Model file for the job. Use its own axes, mm. A direction names the side the tool comes from. Coordinates: 2 decimals unless noted, no trailing zeros. Order: outer loops, then holes, each group sorted by start corner. A loop starts at its lowest first (then second) coordinate and runs counter-clockwise, first axis right, second up. Notation, with made-up numbers: (34.25, 31) -> (80.25, 31) arc R14 ccw to (80.25, 41) -> close; hole circle Ø6 at (58, -29.75). An arc over 180 degrees is marked (long way). Use CSV: the item, a comma, the result in double quotes. Start each with the question number.
(1) Pin check, flat tips, straight feed: pin 1 Ø1.6 at (y, z) = (0, 7.5) entering from -X; pin 2 Ø1 at (x, y) = (-5, -0.5) entering from -Z; pin 3 Ø1.5 at (x, y) = (-21, 0.5) entering from -Z. Stop position of each tip, or through.
(2) Cut at B-B on z = -8. Write the cut outline in (x, y), plus the area to 3 significant figures.
(3) Pull direction X, two halves, no side cores. Call faces 1 (the flat face through (-31, 0, 36.82)), 2 (the flat face through (-38, 0, -33.846)), 3 (the flat face through (-40, 0, 37)): pulls with the +X half, pulls with the -X half, needs draft (parallel to the pull), parting line crosses it, or undercut.
(4) Cut at A-A on x = 20. Write the cut outline in (y, z).
(5) Probe L1, parallel to Z at x = 16.5, y = 0.2. List the from-to ranges inside material, lowest first.
(6) Tool access for faces 4 (the flat face through (-36.82, 0, 6)), 5 (the flat face through (36.82, 0, 31)), 6 (the flat face through (-27.692, 0, 38)), 7 (the flat face through (-18, 0, -36.82)), 8 (the flat face through (0, 0, -40)): list every direction of +Z, -Z, +X, -X, +Y, -Y with a clear straight run to the whole face (end or side of a thin tool).
```python
from build123d import *

# Parameters (mm, degrees)
SKETCH1_W           = 80
SKETCH1_H           = 80
BOSS_EXTRUDE1_DEPTH = 1.5875
SKETCH2_OUTSIDE_W   = 104.636
SKETCH2_OUTSIDE_H   = 104.636
CUT_EXTRUDE1_DEPTH  = 57.657573413


with BuildPart() as part:
    # Sketch1 → Boss-Extrude1 (new, symmetric)
    with BuildSketch(Plane(origin=(0, 0, 0), x_dir=(1, 0, 0), z_dir=(0, 1, 0))):
        Rectangle(SKETCH1_W, SKETCH1_H)
    extrude(amount=BOSS_EXTRUDE1_DEPTH, both=True)

    # Sketch2 outside → Cut-Extrude1 (cut, through all)
    with BuildSketch(Plane(origin=(0, 1.5875, 0), x_dir=(1, 0, 0), z_dir=(0, 1, 0))):
        Rectangle(SKETCH2_OUTSIDE_W, SKETCH2_OUTSIDE_H)
        Polygon((-40, 40), (-40, 33.846153846), (-36.82, 33.846153846), (-36.82, 27.692307692), (-40, 27.692307692), (-40, 21.538461538), (-36.82, 21.538461538), (-36.82, 15.384615385), (-40, 15.384615385), (-40, 9.230769231), (-36.82, 9.230769231), (-36.82, 3.076923077), (-40, 3.076923077), (-40, -3.076923077), (-36.82, -3.076923077), (-36.82, -9.230769231), (-40, -9.230769231), (-40, -15.384615385), (-36.82, -15.384615385), (-36.82, -21.538461538), (-40, -21.538461538), (-40, -27.692307692), (-36.82, -27.692307692), (-36.82, -33.846153846), (-40, -33.846153846), (-40, -40), (-33.846153846, -40), (-33.846153846, -36.82), (-27.692307692, -36.82), (-27.692307692, -40), (-21.538461538, -40), (-21.538461538, -36.82), (-15.384615385, -36.82), (-15.384615385, -40), (-9.230769231, -40), (-9.230769231, -36.82), (-3.076923077, -36.82), (-3.076923077, -40), (3.076923077, -40), (3.076923077, -36.82), (9.230769231, -36.82), (9.230769231, -40), (15.384615385, -40), (15.384615385, -36.82), (21.538461538, -36.82), (21.538461538, -40), (27.692307692, -40), (27.692307692, -36.82), (33.846153846, -36.82), (33.846153846, -40), (40, -40), (40, -33.846153846), (36.82, -33.846153846), (36.82, -27.692307692), (40, -27.692307692), (40, -21.538461538), (36.82, -21.538461538), (36.82, -15.384615385), (40, -15.384615385), (40, -9.230769231), (36.82, -9.230769231), (36.82, -3.076923077), (40, -3.076923077), (40, 3.076923077), (36.82, 3.076923077), (36.82, 9.230769231), (40, 9.230769231), (40, 15.384615385), (36.82, 15.384615385), (36.82, 21.538461538), (40, 21.538461538), (40, 27.692307692), (36.82, 27.692307692), (36.82, 33.846153846), (40, 33.846153846), (40, 40), (33.846153846, 40), (33.846153846, 36.82), (27.692307692, 36.82), (27.692307692, 40), (21.538461538, 40), (21.538461538, 36.82), (15.384615385, 36.82), (15.384615385, 40), (9.230769231, 40), (9.230769231, 36.82), (3.076923077, 36.82), (3.076923077, 40), (-3.076923077, 40), (-3.076923077, 36.82), (-9.230769231, 36.82), (-9.230769231, 40), (-15.384615385, 40), (-15.384615385, 36.82), (-21.538461538, 36.82), (-21.538461538, 40), (-27.692307692, 40), (-27.692307692, 36.82), (-33.846153846, 36.82), (-33.846153846, 40), align=None, mode=Mode.SUBTRACT)
    extrude(amount=-CUT_EXTRUDE1_DEPTH, mode=Mode.SUBTRACT)


solid = part.part
```
Outcome:
1,pin 1,"x = -36.82"
1,pin 2,"z = -36.82"
1,pin 3,"z = -40"
2,outline,"(-36.82, -1.59) -> (36.82, -1.59) -> (36.82, 1.59) -> (-36.82, 1.59) -> close"
2,area,"234 mm2"
3,face 1,"undercut"
3,face 2,"needs draft"
3,face 3,"pulls with the -X half"
4,outline,"(-1.59, -36.82) -> (1.59, -36.82) -> (1.59, 36.82) -> (-1.59, 36.82) -> close"
5,L1,"-36.82 to 36.82"
6,face 4,"-X, +Y, -Y"
6,face 5,"+X, +Y, -Y"
6,face 6,"+Z, +Y, -Y"
6,face 7,"-Z, +Y, -Y"
6,face 8,"-Z, +X, -X, +Y, -Y"
